Print and shaded views of the part. All mm, measured from the part's lowest x, y and z. Coordinates: 2 decimals unless noted, no trailing zeros. Loops run counter-clockwise (first coordinate to the right, second up) from the corner with the lowest first, then second, coordinate; pieces in that order, holes last. Notation, with made-up numbers: (81.25, 59) -> (126.25, 59) arc R19 ccw to (126.25, 79) -> close; hole circle Ø7 at (73.5, 65.25). An arc over 180 degrees is marked (long way). One line per question, with ' | ' between items. Start each with the question number.
1) Cut at A-A (x = 3). List the corners of the cut face in (y, z).
2) Cut at B-B (x = 21). List the corners of the cut face in (y, z) (3 decimals).
3) Drop flat-ended pins along their axis: pin 1 (8 mm diameter, centred on x = 15, z = 5, fed in from +Y); pin 2 (1.5 mm diameter, centred on x = 21.5, y = 23.5, fed in from +Z); pin 3 (2.5 mm diameter, centred on x = 38.5, y = 15.975, fed in from +Z); pin 4 (1.5 mm diameter, centred on y = 14.5, z = 18, fed in from +X). Give the stop position or say it passes through.
4) Cut at C-C (z = 9.25). List the corners of the cut face in (x, y) (3 decimals), plus the area to 3 significant figures.
5) Cut at D-D (y = 25.5). List the corners of the cut face in (x, z).
6) Probe L1, parallel to Y at x = 38.5, z = 18.4 (3 decimals); L2, parallel to Z at x = 30.5, y = 20.5; L3, parallel to X at y = 19.5, z = 11.25. List the from-to ranges inside material, lowest first. Write a range as from..to.
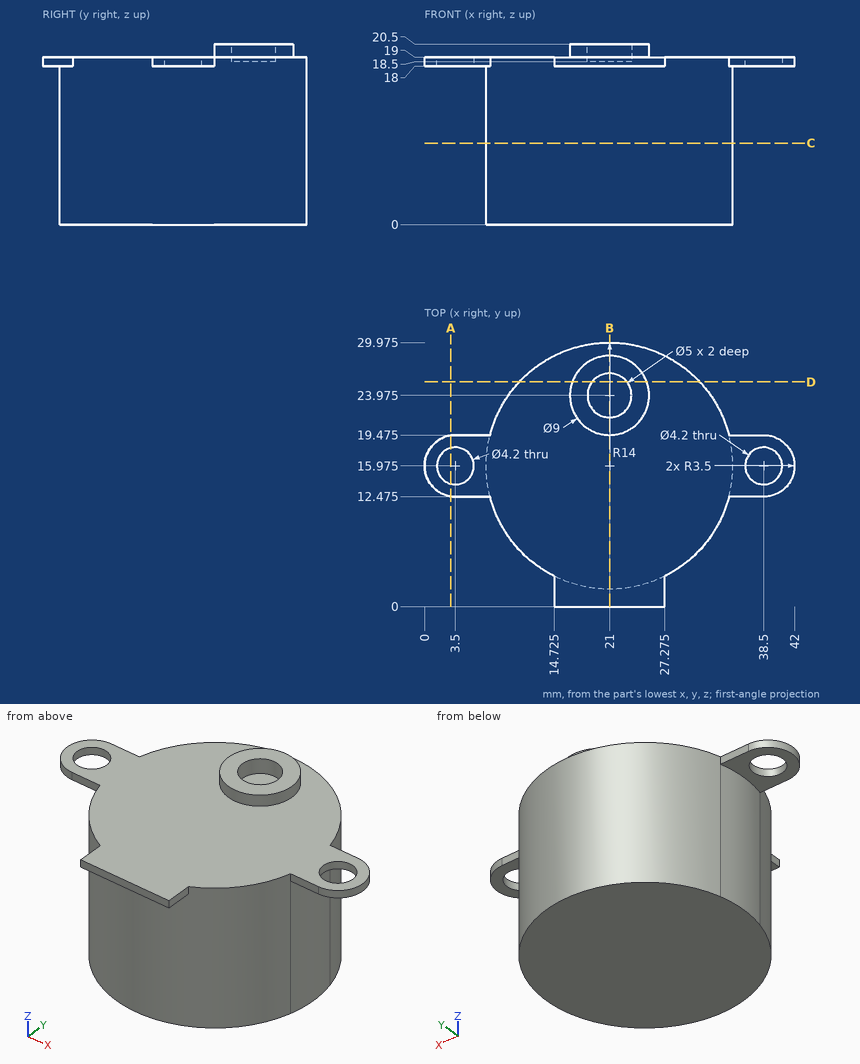
Reported:
1) outline: (12.51, 18) -> (13.94, 18) -> (13.94, 19) -> (12.51, 19) -> close; (18.01, 18) -> (19.44, 18) -> (19.44, 19) -> (18.01, 19) -> close
2) outline: (0, 18) -> (1.975, 18) -> (1.975, 0) -> (29.975, 0) -> (29.975, 19) -> (28.475, 19) -> (28.475, 20.5) -> (26.475, 20.5) -> (26.475, 18.5) -> (21.475, 18.5) -> (21.475, 20.5) -> (19.475, 20.5) -> (19.475, 19) -> (0, 19) -> close
3) pin 1: stops at y = 29.83 | pin 2: stops at z = 18.5 | pin 3: passes through | pin 4: stops at x = 41.92
4) outline: circle Ø28 at (21, 15.975) | area: 616 mm²
5) outline: (10.74, 0) -> (31.26, 0) -> (31.26, 19) -> (25.23, 19) -> (25.23, 20.5) -> (22.98, 20.5) -> (22.98, 18.5) -> (19.02, 18.5) -> (19.02, 20.5) -> (16.77, 20.5) -> (16.77, 19) -> (10.74, 19) -> close
6) L1: y = 12.475..13.875, 18.075..19.475 | L2: z = 0..19 | L3: x = 7.45..34.55
